Print and shaded views of the part. All mm, measured from the part's lowest x, y and z. Round coordinates to 2 decimals unless told otherwise and drop trailing zeros. Write each loop counter-clockwise with the first axis right and the second up, starting at its lowest first coordinate (ties: lowest second). Pieces come first, ordered by that corner, then holes. Notation, with made-up numbers: M 0.5,83.5 L 49.5,83.5 A17 cw 49.5,105.5 Z; hole C 11,64.25 d2. An arc over 180 degrees is marked long. Write item = value, one per line.
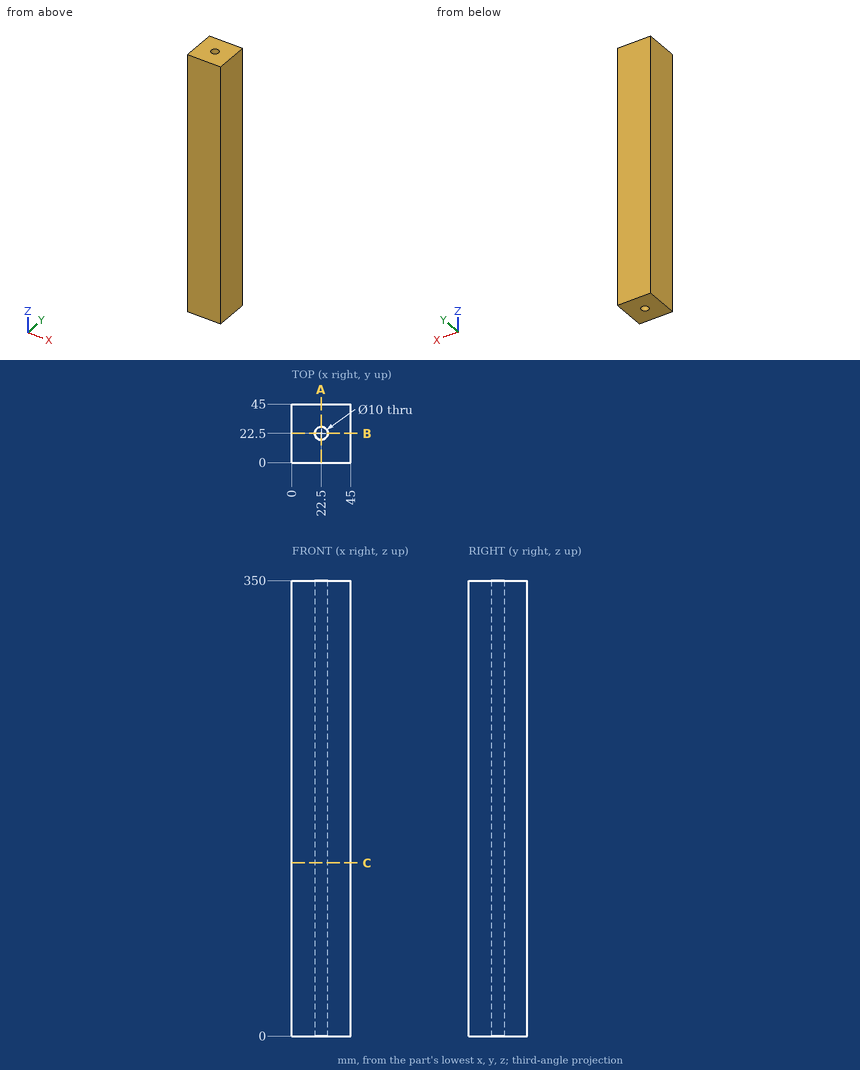
1. Band-saw the part on A-A (x = 22.5). List the corners of the cut face in (y, z), plus the area to 4 significant figures.
Responses:
outline = M 0,0 L 17.5,0 L 17.5,350 L 0,350 Z; M 27.5,0 L 45,0 L 45,350 L 27.5,350 Z
area = 12,250 mm²
2. Flat gauge pin, fed straight in: pin 1 (11.5 mm diameter, centred on x = 22.5, y = 22.5, fed in from +Z). Where does the tip first touch, or does it go through?
Responses:
pin_1 = 350
3. Band-saw the part on C-C (z = 133). List the corners of the cut face in (x, y), plus the area to 3 significant figures.
Responses:
outline = M 0,0 L 45,0 L 45,45 L 0,45 Z; hole C 22.5,22.5 d10
area = 1,950 mm²
4. Probe probe 1 along X at (y, z) = (22, 246); probe 2 along Y at (x, z) = (22.5, 120.5); probe 3 along X at (y, z) = (18, 105). List the from-to ranges inside material, lowest first.
Responses:
probe_1 = 0 to 17.53, 27.47 to 45
probe_2 = 0 to 17.5, 27.5 to 45
probe_3 = 0 to 20.32, 24.68 to 45
